```python
from build123d import *

# Parameters (mm, degrees)
F0_R      = 3.25
F0_R_2    = 1.5
F1_DEPTH  = 10
F2_R      = 5
F3_DEPTH  = 2
F3_FACE_R = 1.5
F4_DEPTH  = 25


with BuildPart() as f1:
    # F0 (on Top) → F1 (new body)
    with BuildSketch(Plane.XY):
        Circle(F0_R)
        Circle(F0_R_2, mode=Mode.SUBTRACT)
    extrude(amount=F1_DEPTH)

    # F2 (on Top) → F3 (join)
    with BuildSketch(Plane.XY):
        Circle(F2_R)
    extrude(amount=F3_DEPTH)

    # F3_face (on face) → F4 (cut)
    with BuildSketch(Plane.XY.offset(2)):
        Circle(F3_FACE_R)
    extrude(amount=-F4_DEPTH, mode=Mode.SUBTRACT)


solid = f1.part
```
For this review, take the finished solid that the model builds, in its own axes (mm). A direction names the side the tool comes from. Give positions to 0.01 mm unless a question says otherwise; leave off trailing zeros. Write each loop counter-clockwise with the first axis right and the second up, starting at its lowest first coordinate (ties: lowest second). Pieces come first, ordered by that corner, then holes.
Item 1: Take a section at B-B (x = -0.5). Give the boundary of the cut face in (y, z), and give its area (3 significant figures).
Item 2: Take a section at A-A (y = 0). Give the boundary of the cut face in (x, z).
Item 3: Insertion check: P1, Ø4, axis at x = -3, z = 5.5, coming from the -Y side; P2, Ø4, axis at y = 4, z = 2, coming from the -X side. Each pin has a flat end and moves straight along its axis. Give the tip position at first contact, or say it passes through.
Item 4: Machinability: for faces 4 (the face through (-1.5, 0.07, 5.07)), 5 (the face through (1, -3.3, 2)), which of the approach directions +Z, -Z, +X, -X, +Y, -Y give a long, thin tool a straight path to every point of the face, cutting with its end or side? Answer none if there is none.
Item 5: Take a section at D-D (y = 2). Give the boundary of the cut face in (x, z), and give its area (3 significant figures).
Item 6: Take a section at C-C (z = 2.25). Give the boundary of the cut face in (x, y), and give its area (3 significant figures).
Item 7: Wall thickness on probe 1 along Y at (x, z) = (0, 5.25); probe 2 along Y at (x, z) = (-1.25, 1); probe 3 along Z at (x, y) = (1.75, 3.5): over which ranges is each line inside the solid? List them lowest first.
Item 8: The part is to be moulded in two halves that separate along Z. For faces 1 (the face through (-1.2, 1.2, 0)), 2 (the face through (-2.579, -1.978, 5.944)), 3 (the face through (0.7, 1.5, 10)), say which applies: +Z half, -Z half, draft (parallel to the pull), parting line (faces both ways), or undercut.
Established:
1. outline: (-4.97, 0) - (-1.41, 0) - (-1.41, 10) - (-3.21, 10) - (-3.21, 2) - (-4.97, 2) - close; (1.41, 0) - (4.97, 0) - (4.97, 2) - (3.21, 2) - (3.21, 10) - (1.41, 10) - close
1. area: 43.0 mm2
2. outline: (-5, 0) - (-1.5, 0) - (-1.5, 10) - (-3.25, 10) - (-3.25, 2) - (-5, 2) - close; (1.5, 0) - (5, 0) - (5, 2) - (3.25, 2) - (3.25, 10) - (1.5, 10) - close
3. P1: stops at y = -3.09
3. P2: stops at x = -4.58
4. face 4: +Z, -Z
4. face 5: +Z
5. outline: (-4.58, 0) - (4.58, 0) - (4.58, 2) - (2.56, 2) - (2.56, 10) - (-2.56, 10) - (-2.56, 2) - (-4.58, 2) - close
5. area: 59.3 mm2
6. outline: circle Ø6.5 at (0, 0); hole circle Ø3 at (0, 0)
6. area: 26.1 mm2
7. probe 1: y = -3.25 to -1.5, 1.5 to 3.25
7. probe 2: y = -4.84 to -0.83, 0.83 to 4.84
7. probe 3: z = 0 to 2
8. face 1: -Z half
8. face 2: draft
8. face 3: +Z half
